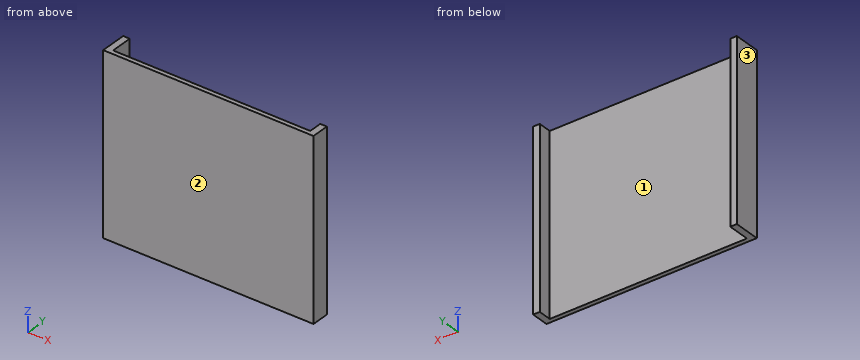
```python
from build123d import *

# Parameters (mm, degrees)
SK_P01_TRAY_W      = 96
SK_P01_TRAY_H      = 81
P01_TRAY_DEPTH     = 2
P02_REARSTOP_START = 2
SK_P02_REARSTOP_W  = 3
SK_P02_REARSTOP_H  = 81
P02_REARSTOP_DEPTH = 10
P03_FRONTLIP_START = 2
SK_P03_FRONTLIP_W  = 3
SK_P03_FRONTLIP_H  = 81
P03_FRONTLIP_DEPTH = 6


with BuildPart() as part:
    # SK_P01_Tray → P01_Tray (new body)
    with BuildSketch(Plane(origin=(0, 0, 0), x_dir=(1, 0, 0), z_dir=(0, 1, 0))):
        Rectangle(SK_P01_TRAY_W, SK_P01_TRAY_H)
    extrude(amount=P01_TRAY_DEPTH)

    # SK_P02_Rearstop → P02_Rearstop (add)
    with BuildSketch(Plane(origin=(0, 0, 0), x_dir=(1, 0, 0), z_dir=(0, 1, 0)).offset(P02_REARSTOP_START)):
        with Locations((-46.5, 0)):
            Rectangle(SK_P02_REARSTOP_W, SK_P02_REARSTOP_H)
    extrude(amount=P02_REARSTOP_DEPTH)

    # SK_P03_Frontlip → P03_Frontlip (add)
    with BuildSketch(Plane(origin=(0, 0, 0), x_dir=(1, 0, 0), z_dir=(0, 1, 0)).offset(P03_FRONTLIP_START)):
        with Locations((46.5, 0)):
            Rectangle(SK_P03_FRONTLIP_W, SK_P03_FRONTLIP_H)
    extrude(amount=P03_FRONTLIP_DEPTH)


solid = part.part
```
Verification items for the finished model (mm, model axes). Face numbers are marked on the shaded views. Give positions to 0.01 mm unless a question says otherwise; leave off trailing zeros. Order: outer loops, then holes, each group sorted by start corner. A loop starts at its lowest first (then second) coordinate and runs counter-clockwise, first axis right, second up. Notation, with made-up numbers: M -31,10.5 L -24,10.5 A25 ccw -24,46.5 Z; hole C -26.5,21.25 d3. An arc over 180 degrees is marked long. Return JSON: item names as keys, results as strings. Group by question number.
1) Section check A-A on y = 5. Record the cut outline in (x, z).
2) Mould release check, pull along X, two halves, no side actions. Record for the marked faces 1, 2 and 3: pulls with the +X half, pulls with the -X half, needs draft (parallel to the pull), parting line crosses it, or undercut.
3) Go/stop test with flat-tipped pins: pin 1 Ø1 at (x, z) = (-37.5, 16.5) entering from +Y; pin 2 Ø10 at (x, z) = (-15.5, -22.5) entering from -Y; pin 3 Ø3.5 at (x, z) = (46.5, 4) entering from +Y. Record where each tip stops, or that it passes through.
4) Section check C-C on x = 29. Record the cut outline in (y, z).
5) Section check B-B on z = -30.5. Record the cut outline in (x, y).
6) Scan lines: line 1 (X direction, y = 5.25, z = -1.5); line 2 (X direction, y = 9, z = 15.5); line 3 (Y direction, x = -1, z = -10.5). Record each from-to range of solid material in increasing order.
Answer block:
{
 "1": {"outline": "M -48,-40.5 L -45,-40.5 L -45,40.5 L -48,40.5 Z; M 45,-40.5 L 48,-40.5 L 48,40.5 L 45,40.5 Z"},
 "2": {"face 1": "undercut", "face 2": "needs draft", "face 3": "pulls with the -X half"},
 "3": {"pin 1": "stops at y = 2", "pin 2": "stops at y = 0", "pin 3": "stops at y = 8"},
 "4": {"outline": "M 0,-40.5 L 2,-40.5 L 2,40.5 L 0,40.5 Z"},
 "5": {"outline": "M -48,0 L 48,0 L 48,8 L 45,8 L 45,2 L -45,2 L -45,12 L -48,12 Z"},
 "6": {"line 1": "x = -48 to -45, 45 to 48", "line 2": "x = -48 to -45", "line 3": "y = 0 to 2"}
}
